Here's how the part is built. I have some questions about the finished solid (model axes, mm). A direction names the side the tool comes from. Give positions to 0.01 mm unless a question says otherwise; leave off trailing zeros. Loops run counter-clockwise (first coordinate to the right, second up) from the corner with the lowest first, then second, coordinate; pieces in that order, holes last.
Q1. If we section it at A-A (x = 11.5): Please give me the cut outline in (y, z), plus the area to 3 significant figures.
Q2. We'd pull the mould along X, two halves only. Please class faces 4 (the face through (36, -5, 6.619)), 5 (the face through (20.385, -12, 0)), 6 (the face through (34.23, -4.583, 12.455)): +X half, -X half, draft (parallel to the pull), parting line (faces both ways), or undercut.
Q3. Will these pins go through, and if not, where does the flat tip stop? P1, Ø4, axis at y = -17, z = -11, coming from the +X side; P2, Ø10.5, axis at x = 33, z = 0, coming from the -Y side; P3, Ø1.5, axis at x = 19.5, y = -8, coming from the +Z side; P4, Ø8, axis at y = -5, z = -1, coming from the +X side.
Q4. I need wall thicknesses on line 1 (Y direction, x = -2, z = -7.5); line 2 (X direction, y = -5.75, z = 7.25); line 3 (X direction, y = -12.5, z = -6.25). Which ranges of each line are inside material? Lowest first, please.
Q5. If we section it at B-B (z = 7.5): Give the number of separate pieces and of enclosed holes in the cut face, plus the area to 3 significant figures.
Q6. For faces 1 (the face through (-20.615, -8, 0)), 2 (the face through (36, -5, -7.881)), 3 (the face through (-26.111, -23.574, 0.003)), which set-ups out of +Z, -Z, +X, -X, +Y, -Y let a thin tool reach every point of the face, with its end or its side?
Q7. If we section it at D-D (y = -21.5): Please give me the cut outline in (x, z).
from build123d import *

# Parameters (mm, degrees)
F0_W           = 41
F0_H           = 27
F1_DEPTH       = 5
F0_W_2         = 7
F2_DEPTH       = 20
F3_DEPTH       = 20
F4_DEPTH       = 10
F5_R           = 2
F8_D           = 3
F8_DEPTH       = 12
F8_TIP         = 0.9012909285
F8_ON_F6_D     = 3
F8_ON_F6_DEPTH = 12
F8_ON_F6_TIP   = 0.9012909285
F9_W           = 48.1226687921
F9_H           = 27
F9_W_2         = 55.1226687921
F10_DEPTH      = 5
F11_R          = 4.99999
F12_W          = 4.2837616056
F12_H          = 27.1169293898
F13_DEPTH      = 4
F14_F1_R       = 1
F14_F2_R       = 1
F15_R          = 1


# Not quite as in the source:
# - a fillet or chamfer is up to 0.001 mm smaller than in the source, because OpenCascade refuses the exact size


with BuildPart() as f1:
    # F0 (on Front) → F1 (new body)
    with BuildSketch(Plane.XZ):
        with Locations((-0.1147079957, -0.1861773429)):
            Rectangle(F0_W, F0_H)
    extrude(amount=F1_DEPTH)

    # F0 (on Front) → F2 (join)
    with BuildSketch(Plane.XZ):
        with Locations((23.8852920043, -0.1861773429)):
            Rectangle(F0_W_2, F0_H)
    extrude(amount=F2_DEPTH)

    # F0 (on Front) → F3 (join)
    with BuildSketch(Plane.XZ):
        with Locations((-24.1147079957, -0.1861773429)):
            Rectangle(F0_W_2, F0_H)
    extrude(amount=F3_DEPTH)

    # F0 (on Front) → F4 (join)
    with BuildSketch(Plane.XZ):
        Polygon((40.8852920043, 11.6193783459), (27.3852920043, 13.3138226571), (27.3852920043, -13.6861773429), (40.8852920043, -12.8806216541), (40.8852920043, -7.8806216541), (32.3852920043, -7.8806216541), (32.3852920043, 6.6193783459), (40.8852920043, 6.6193783459), align=None)
    extrude(amount=F4_DEPTH)

    # F5
    f5_edges = [f1.edges().sort_by_distance(p)[0] for p in [
        (27.385292, -10, -0.186177),
        (-27.614708, 0, -0.186177),
        (40.885292, -10, -10.380622),
        (40.885292, -10, 9.119378),
    ]]
    fillet(f5_edges, radius=F5_R)

    # F8 (one way)
    with BuildSketch(Plane(origin=(0, 0, 6.6193783459), x_dir=(1, 0, 0), z_dir=(0, 0, -1))):
        with Locations((37.8852920043, 5)):
            Circle(F8_D / 2)
    extrude(amount=-F8_DEPTH, mode=Mode.SUBTRACT)
    with Locations(Plane(origin=(0, 0, 6.6193783459), x_dir=(1, 0, 0), z_dir=(0, 0, -1))):
        with Locations((37.8852920043, 5)):
            with Locations((0, 0, -(F8_DEPTH + F8_TIP / 2))):  # 118° drill point
                Cone(0, F8_D / 2, F8_TIP, mode=Mode.SUBTRACT)

    # F8 on F6 (one way)
    with BuildSketch(Plane.XY.offset(-7.8806216541)):
        with Locations((37.8852920043, -5)):
            Circle(F8_ON_F6_D / 2)
    extrude(amount=-F8_ON_F6_DEPTH, mode=Mode.SUBTRACT)
    with Locations(Plane.XY.offset(-7.8806216541)):
        with Locations((37.8852920043, -5)):
            with Locations((0, 0, -(F8_ON_F6_DEPTH + F8_ON_F6_TIP / 2))):  # 118° drill point
                Cone(0, F8_ON_F6_D / 2, F8_ON_F6_TIP, mode=Mode.SUBTRACT)

    # F9 (on face) → F10 (join)
    with BuildSketch(Plane.XZ.offset(20)):
        with Locations((3.4466264003, -0.1861773429)):
            Rectangle(F9_W, F9_H)
        with Locations((-0.0533735997, -0.1861773429)):
            Rectangle(F9_W_2, F9_H)
    extrude(amount=F10_DEPTH)

    # F11 (radius 5 in the source; OpenCascade refuses exactly that, so slightly less here)
    f11_edges = [f1.edges().sort_by_distance(p)[0] for p in [
        (27.507961, -25, -0.186177),
        (-27.614708, -25, -0.186177),
    ]]
    fillet(f11_edges, radius=F11_R)

    # F12 (on face) → F13 (cut)
    with BuildSketch(Plane.YZ.offset(-20.6147079957)):
        with Locations((-12.8439003602, -0.2446420378)):
            Rectangle(F12_W, F12_H)
    extrude(amount=-F13_DEPTH, mode=Mode.SUBTRACT)

    # F14: fillet of radius 1 on 3 edges, made by hand

    # F14_f1
    f14_f1_edges = [f1.edges().sort_by_distance(p)[0] for p in [
        (-24.6147079957, -14.985781163, -0.1861773429),
        (-24.6147079957, -10.7020195574, -0.1861773429),
    ]]
    fillet(f14_f1_edges, radius=F14_F1_R)

    # F14_f2
    f14_f2_edges = [f1.edges().sort_by_distance(p)[0] for p in [
        (-24.6147079957, -12.8439003602, 13.3138226571),
        (-24.3218147769, -10.9949127762, 13.3138226571),
        (-24.3218147769, -14.6928879442, 13.3138226571),
    ]]
    fillet(f14_f2_edges, radius=F14_F2_R)

    # F15
    f15_edges = [f1.edges().sort_by_distance(p)[0] for p in [
        (-22.114708, -14.985781, -13.686177),
        (-22.114708, -10.70202, -13.686177),
        (-24.321815, -10.994913, -13.686177),
        (-24.614708, -12.8439, -13.686177),
        (-24.321815, -14.692888, -13.686177),
    ]]
    fillet(f15_edges, radius=F15_R)


solid = f1.part
Check sheet entries:
1. outline: (-25, -13.69) - (-20, -13.69) - (-20, 13.31) - (-25, 13.31) - close; (-5, -13.69) - (0, -13.69) - (0, 13.31) - (-5, 13.31) - close
1. area: 270 mm2
2. face 4: draft
2. face 5: undercut
2. face 6: +X half
3. P1: stops at x = 27.39
3. P2: stops at y = -10.85
3. P3: passes through
3. P4: stops at x = 32.39
4. line 1: y = -25 to -20, -5 to 0
4. line 2: x = -27.61 to -20.61, 20.39 to 36.59, 39.18 to 40.89
4. line 3: x = -27.61 to -24.61, 20.39 to 27.39
5. separate pieces: 1
5. enclosed holes: 2
5. area: 860 mm2
6. face 1: +Z, -Z
6. face 2: +X, +Y, -Y
6. face 3: +Z, -Z, -X, -Y
7. outline: (-27.38, -13.69) - (27.28, -13.69) - (27.28, 13.31) - (-27.38, 13.31) - close
